Read the model definition and answer for the solid it produces. Units are mm, in the model's axes. Face numbers are marked on the shaded views. A direction names the side the tool comes from. Coordinates: 2 decimals unless noted, no trailing zeros. Order: outer loops, then holes, each group sorted by start corner. A loop starts at its lowest first (then second) coordinate and runs counter-clockwise, first axis right, second up.
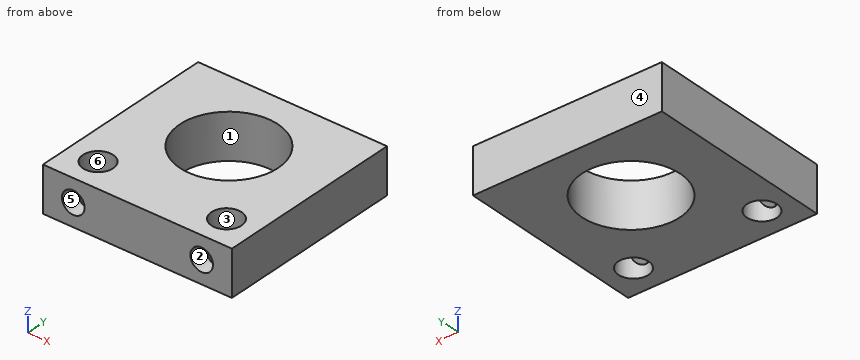
```python
from build123d import *

# Parameters (mm, degrees)
SKETCH1_W           = 50
SKETCH1_H           = 50
BOSS_EXTRUDE1_DEPTH = 12
CUT_EXTRUDE1_REACH  = 39.336
SKETCH2_R           = 13
CUT_EXTRUDE2_REACH  = 39.336
SKETCH3_R           = 4
CUT_EXTRUDE3_REACH  = 59.175
SKETCH4_R           = 3


with BuildPart() as part:
    # Sketch1 → Boss-Extrude1 (new body)
    with BuildSketch(Plane.XY):
        Rectangle(SKETCH1_W, SKETCH1_H)
    extrude(amount=BOSS_EXTRUDE1_DEPTH)

    # Sketch2 → Cut-Extrude1 (cut, up to next)
    with BuildSketch(Plane.XY.offset(12), mode=Mode.PRIVATE) as cut_extrude1_sk1:
        with Locations((0, 4.5)):
            Circle(SKETCH2_R)
    cut_extrude1_tool1 = extrude(cut_extrude1_sk1.sketch, amount=-CUT_EXTRUDE1_REACH, mode=Mode.PRIVATE) & part.part
    add(cut_extrude1_tool1.solids().sort_by_distance((0, 4.5, 12))[0], mode=Mode.SUBTRACT)

    # Sketch3 → Cut-Extrude2 (cut, up to next)
    with BuildSketch(Plane.XY.offset(12), mode=Mode.PRIVATE) as cut_extrude2_sk1:
        with Locations((-17, -17)):
            Circle(SKETCH3_R)
    cut_extrude2_tool1 = extrude(cut_extrude2_sk1.sketch, amount=-CUT_EXTRUDE2_REACH, mode=Mode.PRIVATE) & part.part
    # Sketch3 → Cut-Extrude2 (cut, up to next)
    with BuildSketch(Plane.XY.offset(12), mode=Mode.PRIVATE) as cut_extrude2_sk2:
        with Locations((17, -17)):
            Circle(SKETCH3_R)
    cut_extrude2_tool2 = extrude(cut_extrude2_sk2.sketch, amount=-CUT_EXTRUDE2_REACH, mode=Mode.PRIVATE) & part.part
    add(cut_extrude2_tool1.solids().sort_by_distance((-17, -17, 12))[0], mode=Mode.SUBTRACT)
    add(cut_extrude2_tool2.solids().sort_by_distance((17, -17, 12))[0], mode=Mode.SUBTRACT)

    # Sketch4 → Cut-Extrude3 (cut, up to next)
    with BuildSketch(Plane.XZ.offset(25), mode=Mode.PRIVATE) as cut_extrude3_sk1:
        with Locations(Location((17, 6, 0), (0, 0, 270))):
            Circle(SKETCH4_R)
    cut_extrude3_tool1 = extrude(cut_extrude3_sk1.sketch, amount=-CUT_EXTRUDE3_REACH, mode=Mode.PRIVATE) & part.part
    # Sketch4 → Cut-Extrude3 (cut, up to next)
    with BuildSketch(Plane.XZ.offset(25), mode=Mode.PRIVATE) as cut_extrude3_sk2:
        with Locations(Location((-17, 6, 0), (0, 0, 270))):
            Circle(SKETCH4_R)
    cut_extrude3_tool2 = extrude(cut_extrude3_sk2.sketch, amount=-CUT_EXTRUDE3_REACH, mode=Mode.PRIVATE) & part.part
    add(cut_extrude3_tool1.solids().sort_by_distance((17, -25, 6))[0], mode=Mode.SUBTRACT)
    add(cut_extrude3_tool2.solids().sort_by_distance((-17, -25, 6))[0], mode=Mode.SUBTRACT)


solid = part.part
```
1) A cutting plane is placed at C-C, the plane z = 6. Determine the outline of the cut face in (x, y), and give its area (3 significant figures).
A:
outline: (-25, -25) - (-20, -25) - (-20, -19.65) arc R4 cw (long way) to (-14, -19.65) - (-14, -25) - (14, -25) - (14, -19.65) arc R4 cw (long way) to (20, -19.65) - (20, -25) - (25, -25) - (25, 25) - (-25, 25) - close; hole circle Ø26 at (0, 4.5)
area: 1,820 mm2
2) Determine the mould class of the marked faces 1, 2, 3 and 4 for opening direction Y: pulls with the +Y half, pulls with the -Y half, needs draft (parallel to the pull), parting line crosses it, or undercut.
A:
face 1: undercut
face 2: needs draft
face 3: undercut
face 4: pulls with the +Y half
3) A cutting plane is placed at A-A, the plane y = 4.5. Determine the outline of the cut face in (x, z), and give its area (3 significant figures).
A:
outline: (-25, 0) - (-13, 0) - (-13, 12) - (-25, 12) - close; (13, 0) - (25, 0) - (25, 12) - (13, 12) - close
area: 288 mm2
4) A cutting plane is placed at B-B, the plane x = -17. Determine the outline of the cut face in (y, z).
A:
outline: (-25, 0) - (-21, 0) - (-21, 3) - (-25, 3) - close; (-25, 9) - (-21, 9) - (-21, 12) - (-25, 12) - close; (-13, 0) - (25, 0) - (25, 12) - (-13, 12) - close
5) Straight lines are drawn through the part: line 1 (X direction, y = -21.9, z = 6); line 2 (Z direction, x = -17, y = -23.45); line 3 (X direction, y = -20.5, z = 2). For each, find the intervals that lie inside material, in ascending order.
A:
line 1: x = -25 to -20, -14 to 14, 20 to 25
line 2: z = 0 to 3, 9 to 12
line 3: x = -25 to -18.94, -15.06 to 15.06, 18.94 to 25
6) Which of the six approach directions +Z, -Z, +X, -X, +Y, -Y give full straight-line access (tool end or side, diameter ignored) to the marked faces 5 and 6?
A:
face 5: -Y
face 6: +Z, -Z
7) A cutting plane is placed at D-D, the plane x = 0. Determine the outline of the cut face in (y, z), and give its area (3 significant figures).
A:
outline: (-25, 0) - (-8.5, 0) - (-8.5, 12) - (-25, 12) - close; (17.5, 0) - (25, 0) - (25, 12) - (17.5, 12) - close
area: 288 mm2
